from build123d import *

# Parameters (mm, degrees)
F1_DEPTH = 4.445
F2_R     = 2
F2_W     = 6.084966
F2_H     = 4
F3_DEPTH = 25
F4_R     = 3.15
F5_DEPTH = 5
F6_W     = 7.922152
F6_H     = 6
F7_DEPTH = 4


with BuildPart() as f1:
    # F0 (on Top) → F1 (new body, symmetric)
    with BuildSketch(Plane.XY):
        Polygon((-30, 9), (-30, 0), (-18.787624, 0), (-11.558056, 4), (0, 4), (11.558056, 4), (18.787624, 0), (30, 0), (30, 9), (18.787624, 9), (11.558056, 13), (0, 13), (-11.558056, 13), (-18.787624, 9), align=None)
    extrude(amount=F1_DEPTH, both=True)

    # F2 (on face) → F3 (cut)
    with BuildSketch(Plane(origin=(0, 13, 0), x_dir=(-1, 0, 0), z_dir=(0, 1, 0))):
        Circle(F2_R)
        with Locations((-25, 0)):
            Rectangle(F2_W, F2_H)
        with Locations((25, 0)):
            Rectangle(F2_W, F2_H)
    extrude(amount=-F3_DEPTH, mode=Mode.SUBTRACT)

    # F4 (on face) → F5 (cut)
    with BuildSketch(Plane.XZ.offset(-4)):
        Circle(F4_R)
    extrude(amount=-F5_DEPTH, mode=Mode.SUBTRACT)

    # F6 (on face) → F7 (cut)
    with BuildSketch(Plane(origin=(0, 9, 0), x_dir=(-1, 0, 0), z_dir=(0, 1, 0))):
        with Locations((-24.973184, 0)):
            Rectangle(F6_W, F6_H)
        with Locations((24.973184, 0)):
            Rectangle(F6_W, F6_H)
    extrude(amount=-F7_DEPTH, mode=Mode.SUBTRACT)


solid = f1.part
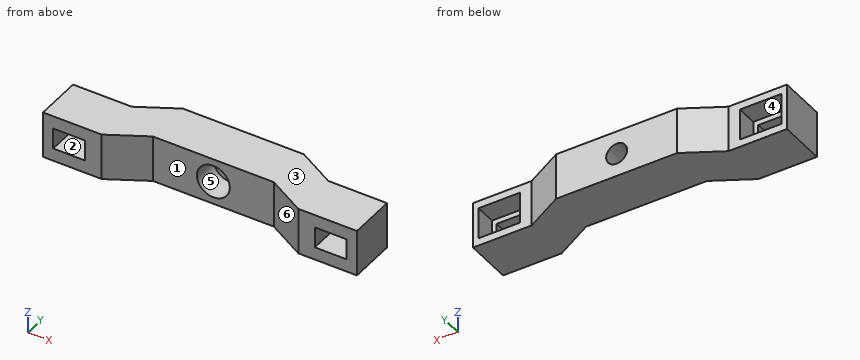
Design review of the part built by this model. Coordinates are the model's own, in mm. Face numbers are marked on the shaded views. A direction names the side the tool comes from. Round coordinates to 2 decimals unless told otherwise and drop trailing zeros. Loops run counter-clockwise (first coordinate to the right, second up) from the corner with the lowest first, then second, coordinate; pieces in that order, holes last. Notation, with made-up numbers: (45.25, -33) -> (83.25, -33) arc R22 ccw to (83.25, -24) -> close; hole circle Ø1 at (37, 48). An arc over 180 degrees is marked (long way). Use one line per item in the form item = value. Start each with the question number.
Q1. We need section B-B on x = 0. Give the boundary of the cut face in (y, z) (3 decimals), then the cut area to 3 significant figures.
Q2. We need section D-D on z = 0. State how many separate pieces and enclosed holes the cut face has, then the cut area to 3 significant figures.
Q3. We need section C-C on y = 6.75. Give the boundary of the cut face in (x, z) (3 decimals).
Q4. Draft analysis for pull direction Z (two halves, no side actions). For the marked faces 1, 2 and 3, state which applies: +Z half, -Z half, draft (parallel to the pull), parting line (faces both ways), or undercut.
Q5. We need section A-A on y = 1. Give the boundary of the cut face in (x, z) (3 decimals).
Q6. For pin 1 Ø4.5 at (x, z) = (-21.5, -1.5) entering from +Y; pin 2 Ø1.5 at (x, z) = (-1, -2.5) entering from -Y; pin 3 Ø5 at (x, z) = (0, 0) entering from -Y, all flat-tipped, find the tip position at first contact; note any pin that passes through.
Q7. Machinability: for the marked faces 4, 5 and 6, which of the approach directions +Z, -Z, +X, -X, +Y, -Y give a long, thin tool a straight path to every point of the face, cutting with its end or side? Answer none if there is none.
Q8. Wall thickness on line 1 along X through (y, z) = (7, 0.25); line 2 along Z through (x, y) = (0, 11.85) (3 decimals); line 3 along Z through (x, y) = (0, 5.3) (3 decimals): over which ranges is each line inside the solid? List them lowest first. Write a range as [from, to].
Calculated:
q1.outline = (4, -4.445) -> (13, -4.445) -> (13, -2) -> (9, -2) -> (9, -3.15) -> (4, -3.15) -> close; (4, 3.15) -> (9, 3.15) -> (9, 2) -> (13, 2) -> (13, 4.445) -> (4, 4.445) -> close
q1.area = 32.5 mm²
q2.separate_pieces = 4
q2.enclosed_holes = 0
q2.area = 368 mm²
q3.outline = (-30, -4.445) -> (30, -4.445) -> (30, 4.445) -> (-30, 4.445) -> close; hole (-28.934, -3) -> (-21.012, -3) -> (-21.012, 3) -> (-28.934, 3) -> close; hole circle Ø6.3 at (0, 0); hole (21.012, -3) -> (28.934, -3) -> (28.934, 3) -> (21.012, 3) -> close
q4.face_1 = draft
q4.face_2 = undercut
q4.face_3 = +Z half
q5.outline = (-30, -4.445) -> (-16.98, -4.445) -> (-16.98, 4.445) -> (-30, 4.445) -> close; (16.98, -4.445) -> (30, -4.445) -> (30, 4.445) -> (16.98, 4.445) -> close; hole (-28.042, -2) -> (-21.958, -2) -> (-21.958, 2) -> (-28.042, 2) -> close; hole (21.958, -2) -> (28.042, -2) -> (28.042, 2) -> (21.958, 2) -> close
q6.pin_1 = 9
q6.pin_2 = 4
q6.pin_3 = 9
q7.face_4 = +Y
q7.face_5 = -Y
q7.face_6 = +Z, -Z, -Y
q8.line_1 = [-30, -28.93], [-21.01, -3.14], [3.14, 21.01], [28.93, 30]
q8.line_2 = [-4.445, -2], [2, 4.445]
q8.line_3 = [-4.445, -3.15], [3.15, 4.445]
